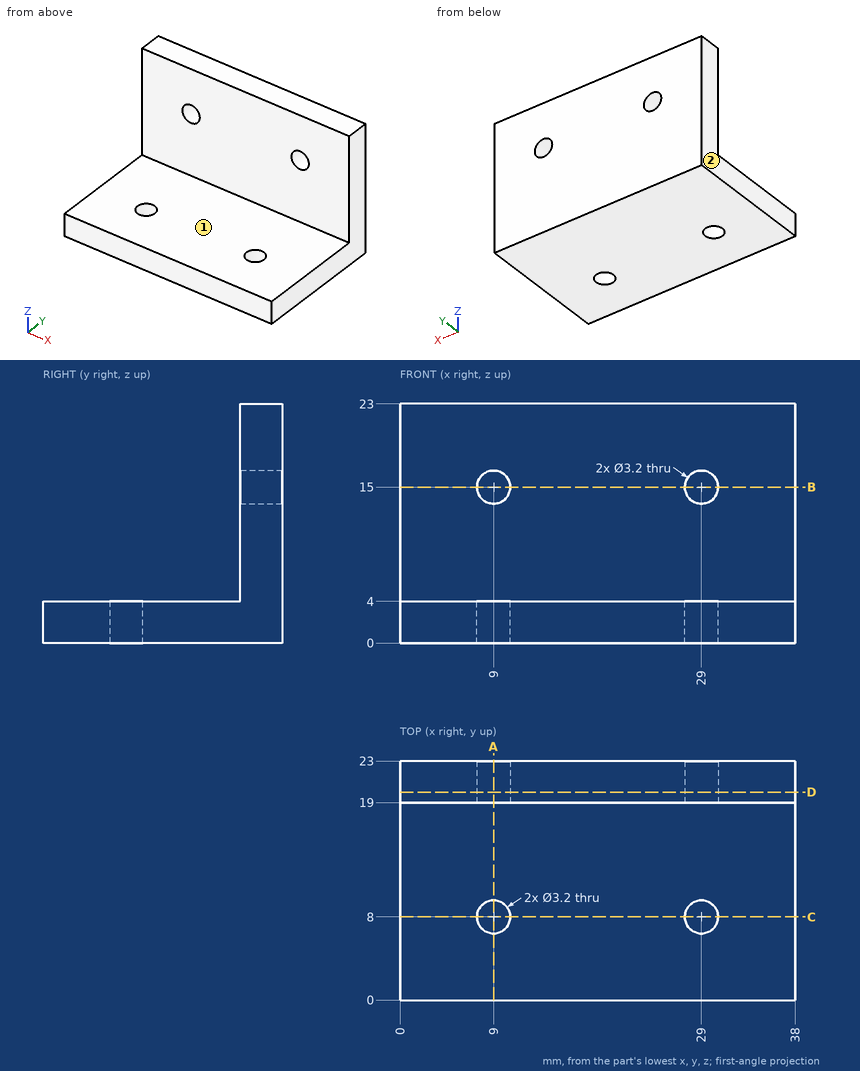
Check sheet for the drawn part. Datum: minimum x, y, z corner. Units: mm. A direction names the side the tool comes from. Coordinates: 2 decimals unless noted, no trailing zeros. Write each loop counter-clockwise with the first axis right and the second up, starting at its lowest first coordinate (ties: lowest second). Pieces come first, ordered by that corner, then holes. Notation, with made-up numbers: (15, 87) - (38, 87) arc R12 cw to (38, 93) - close; hole circle Ø6 at (-18.5, 52.25). An arc over 180 degrees is marked (long way). Answer as a JSON object with one key per item and string values.
(1) Tool access check on the marked faces 1 and 2. Record the directions out of +Z, -Z, +X, -X, +Y, -Y that give a thin tool (end or side, any length) a straight path to the whole face; none if there is none.
Report:
{"face 1": "+Z, +X, -X, -Y", "face 2": "+Z, -Z, -X, +Y, -Y"}
(2) Cross-section at C-C on y = 8. Record the cut outline in (x, z), plus the area to 3 significant figures.
Report:
{"outline": "(0, 0) - (7.4, 0) - (7.4, 4) - (0, 4) - close; (10.6, 0) - (27.4, 0) - (27.4, 4) - (10.6, 4) - close; (30.6, 0) - (38, 0) - (38, 4) - (30.6, 4) - close", "area": "126 mm^2"}
(3) Thickness scan on line 1 along X through (y, z) = (21.6, 15); line 2 along Y through (x, z) = (9, 2.45); line 3 along Z through (x, y) = (9, 20.65). Record the ranges inside material, lowest first.
Report:
{"line 1": "0 to 7.4, 10.6 to 27.4, 30.6 to 38", "line 2": "0 to 6.4, 9.6 to 23", "line 3": "0 to 13.4, 16.6 to 23"}
(4) Cross-section at A-A on x = 9. Record the cut outline in (y, z).
Report:
{"outline": "(0, 0) - (6.4, 0) - (6.4, 4) - (0, 4) - close; (9.6, 0) - (23, 0) - (23, 13.4) - (19, 13.4) - (19, 4) - (9.6, 4) - close; (19, 16.6) - (23, 16.6) - (23, 23) - (19, 23) - close"}
(5) Gauge pin test, flat ends, axial feed: pin 1 Ø5.5 at (x, z) = (23.5, 16.5) entering from -Y; pin 2 Ø2 at (x, y) = (32.5, 3) entering from +Z. Record the tip position at first contact, or that the pin passes through.
Report:
{"pin 1": "y = 19", "pin 2": "z = 4"}
(6) Cross-section at B-B on z = 15. Record the cut outline in (x, y).
Report:
{"outline": "(0, 19) - (7.4, 19) - (7.4, 23) - (0, 23) - close; (10.6, 19) - (27.4, 19) - (27.4, 23) - (10.6, 23) - close; (30.6, 19) - (38, 19) - (38, 23) - (30.6, 23) - close"}
(7) Cross-section at D-D on y = 20. Record the cut outline in (x, z), plus the area to 3 significant figures.
Report:
{"outline": "(0, 0) - (38, 0) - (38, 23) - (0, 23) - close; hole circle Ø3.2 at (9, 15); hole circle Ø3.2 at (29, 15)", "area": "858 mm^2"}
